Model file for the job. Use its own axes, mm. Face numbers are marked on the shaded views. A direction names the side the tool comes from. Round coordinates to 2 decimals unless told otherwise and drop trailing zeros. Loops run counter-clockwise (first coordinate to the right, second up) from the corner with the lowest first, then second, coordinate; pieces in that order, holes last. Notation, with made-up numbers: M 46.25,48.25 L 78.25,48.25 A12 cw 78.25,60.25 Z; hole C 22.5,43.25 d5. An arc over 180 degrees is marked long. Use a Markdown table: item, result. Add a question column.
Q1. Probe line 1 (X direction, y = 10.5, z = -6.25) (3 decimals); line 2 (Y direction, x = 10.5, z = 5.25) (3 decimals); line 3 (Y direction, x = -18.5, z = 3.25) (3 decimals). List the from-to ranges inside material, lowest first. Write a range as from..to.
Q2. Cut at D-D (y = -11.5). Give the cut face in (x, z) (1 decimal), plus the area to 3 significant figures.
Q3. Mould opens along X. For the marked faces 3, 4, 5 and 6 say: +X half, -X half, draft (parallel to the pull), parting line (faces both ways), or undercut.
Q4. Tool access for the marked faces 1 and 2: list every direction of +Z, -Z, +X, -X, +Y, -Y with a clear straight run to the whole face (end or side of a thin tool).
Q5. Cut at C-C (x = 0). Give the cut face in (y, z) (1 decimal), plus the area to 3 significant figures.
Q6. Cut at B-B (x = -13). Give the cut face in (y, z) (1 decimal), plus the area to 3 significant figures.
Q7. Cut at A-A (z = 0). State how many separate pieces and enclosed holes the cut face has, plus the area to 3 significant figures.
Q8. Pin check, flat tips, straight feed: pin 1 (1.9 mm diameter, centred on x = 0, z = 0, fed in from +Y); pin 2 (3 mm diameter, centred on x = -15.875, z = 0, fed in from +Y); pin 3 (4 mm diameter, centred on x = 0, z = 0, fed in from +Y) (3 decimals); pin 4 (6 mm diameter, centred on x = 22, y = -38, fed in from +Z). Stop position of each tip, or through.
from build123d import *

# Parameters (mm, degrees)
F0_W      = 34.925
F0_H      = 52.705
F1_DEPTH  = 10.795
F2_DEPTH  = 10.795
F3_W      = 25.781
F3_H      = 43.18
F3_H_2    = 36.83
F4_DEPTH  = 25.4
F5_R      = 8.255
F6_W      = 34.925
F6_H      = 19.05
F7_DEPTH  = 5.08
F8_R      = 1.5875
F9_DEPTH  = 50.8
F10_R     = 7.493
F11_DEPTH = 76.2
F12_R     = 8.001
F13_R     = 1.5875
F14_DEPTH = 25.4
F15_SIZE  = 0.762
F16_R     = 2.54
F17_SIZE  = 0.8255
F19_W     = 73.3495355977
F19_H     = 43.3503502247
F20_DEPTH = 25.4
F21_R     = 1.5875
F22_DEPTH = 25.4


with BuildPart() as f1:
    # F0 (on Top) → F1 (new body)
    with BuildSketch(Plane.XY):
        with Locations((-17.4625, -26.3525)):
            Rectangle(F0_W, F0_H)
        with Locations((-17.4625, 26.3525)):
            Rectangle(F0_W, F0_H)
        Polygon((0, 52.705), (0, 0), (0, -52.705), (34.925, -52.705), (34.925, 0), (34.925, 52.705), align=None)
    extrude(amount=F1_DEPTH)

    # F0 (on Top) → F2 (join)
    with BuildSketch(Plane.XY):
        with Locations((-17.4625, -26.3525)):
            Rectangle(F0_W, F0_H)
        with Locations((-17.4625, 26.3525)):
            Rectangle(F0_W, F0_H)
        Polygon((0, 52.705), (0, 0), (0, -52.705), (34.925, -52.705), (34.925, 0), (34.925, 52.705), align=None)
    extrude(amount=-F2_DEPTH)

    # F3 (on face) → F4 (cut)
    with BuildSketch(Plane.XY.offset(10.795)):
        with Locations((-12.8905, -21.59)):
            Rectangle(F3_W, F3_H)
        with Locations((-12.8905, 18.415)):
            Rectangle(F3_W, F3_H_2)
        with Locations((12.8905, -21.59)):
            Rectangle(F3_W, F3_H)
        with Locations((12.8905, 18.415)):
            Rectangle(F3_W, F3_H_2)
    extrude(amount=-F4_DEPTH, mode=Mode.SUBTRACT)

    # F5
    f5_edges = [f1.edges().sort_by_distance(p)[0] for p in [
        (-25.781, 36.83, 0),
        (25.781, 36.83, 0),
        (-25.781, -43.18, 0),
        (25.781, -43.18, 0),
    ]]
    fillet(f5_edges, radius=F5_R)

    # F6 (on face) → F7 (join)
    with BuildSketch(Plane(origin=(0, 52.705, 0), x_dir=(-1, 0, 0), z_dir=(0, 1, 0))):
        Polygon((-34.925, 0), (0, 0), (0, -19.05), (34.925, -19.05), (34.925, 0), (34.925, 19.05), (0, 19.05), (-34.925, 19.05), align=None)
        with Locations((-17.4625, -9.525)):
            Rectangle(F6_W, F6_H)
    extrude(amount=-F7_DEPTH)

    # F8 (on face) → F9 (cut)
    with BuildSketch(Plane.XZ.offset(-47.625)):
        with Locations((22.225, 15.24)):
            Circle(F8_R)
        with Locations((0, 15.24)):
            Circle(F8_R)
        with Locations((0, -15.24)):
            Circle(F8_R)
        with Locations((22.225, -15.24)):
            Circle(F8_R)
        with Locations((-22.225, 15.24)):
            Circle(F8_R)
        with Locations((-22.225, -15.24)):
            Circle(F8_R)
    extrude(amount=-F9_DEPTH, mode=Mode.SUBTRACT)

    # F10 (on face) → F11 (cut)
    with BuildSketch(Plane(origin=(-34.925, 0, 0), x_dir=(0, -1, 0), z_dir=(-1, 0, 0))):
        with Locations((-52.705, 0)):
            Circle(F10_R)
    extrude(amount=-F11_DEPTH, mode=Mode.SUBTRACT)

    # F12
    f12_edges = [f1.edges().sort_by_distance(p)[0] for p in [
        (34.925, -52.705, 0),
        (-34.925, -52.705, 0),
    ]]
    fillet(f12_edges, radius=F12_R)

    # F13 (on face) → F14 (cut)
    with BuildSketch(Plane(origin=(0, 52.705, 0), x_dir=(-1, 0, 0), z_dir=(0, 1, 0))):
        Circle(F13_R)
        with Locations((-15.875, 0)):
            Circle(F13_R)
        with Locations((15.875, 0)):
            Circle(F13_R)
    extrude(amount=-F14_DEPTH, mode=Mode.SUBTRACT)

    # F15
    f15_edges = [f1.edges().sort_by_distance(p)[0] for p in [
        (17.4625, 45.212, 0),
        (1.5875, 45.212, 0),
        (-14.2875, 45.212, 0),
    ]]
    chamfer(f15_edges, length=F15_SIZE)

    # F16
    f16_edges = [f1.edges().sort_by_distance(p)[0] for p in [
        (0, 47.625, -10.795),
        (0, 47.625, 10.795),
    ]]
    fillet(f16_edges, radius=F16_R)

    # F17
    f17_edges = [f1.edges().sort_by_distance(p)[0] for p in [
        (25.781, -3.175, 10.795),
        (34.925, 0.1905, 10.795),
        (34.925, 0.1905, -10.795),
        (25.781, -3.175, -10.795),
        (0, 47.625, -19.05),
        (0, 47.625, 19.05),
    ]]
    chamfer(f17_edges, length=F17_SIZE)

    # F19 (on offset) → F20 (cut)
    with BuildSketch(Plane.XZ.offset(-42.545)):
        with Locations((-0.421330399, -0.413473639)):
            Rectangle(F19_W, F19_H)
    extrude(amount=-F20_DEPTH, mode=Mode.SUBTRACT)

    # F21 (on face) → F22 (cut)
    with BuildSketch(Plane.XZ.offset(52.705)):
        Circle(F21_R)
    extrude(amount=-F22_DEPTH, mode=Mode.SUBTRACT)


solid = f1.part
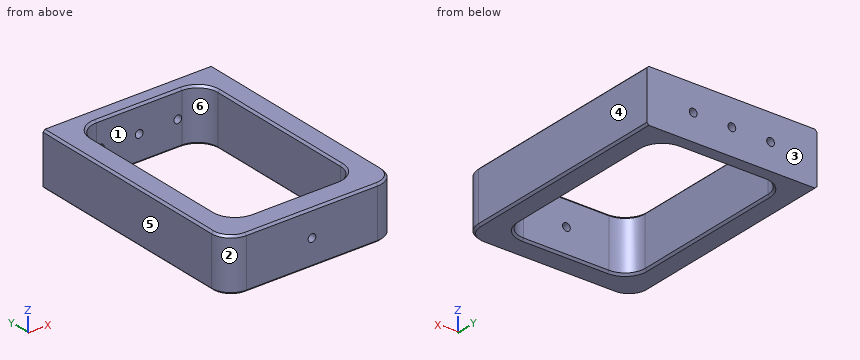
Checked values:
| question | item | result |
|---|---|---|
| 1 | line 1 | x = -34.925..-25.781, 25.781..34.925 |
| 1 | line 2 | y = -52.705..-43.18, 36.83..42.545 |
| 1 | line 3 | y = -52.705..-43.122, 36.772..42.545 |
| 2 | outline | M -34.9,-10 L -34.1,-10.8 L -26.6,-10.8 L -25.8,-10 L -25.8,10 L -26.6,10.8 L -34.1,10.8 L -34.9,10 Z; M 25.8,-10 L 26.6,-10.8 L 34.1,-10.8 L 34.9,-10 L 34.9,10 L 34.1,10.8 L 26.6,10.8 L 25.8,10 Z |
| 2 | area | 392 mm^2 |
| 3 | face 3 | draft |
| 3 | face 4 | +X half |
| 3 | face 5 | -X half |
| 3 | face 6 | undercut |
| 4 | face 1 | +Z, -Z |
| 4 | face 2 | +Z, -Z, -X, -Y |
| 5 | outline | M -52.7,-10 L -51.9,-10.8 L -44,-10.8 L -43.2,-10 L -43.2,-1.6 L -52.7,-1.6 Z; M -52.7,1.6 L -43.2,1.6 L -43.2,10 L -44,10.8 L -51.9,10.8 L -52.7,10 Z; M 36.8,-10 L 37.7,-10.8 L 42.5,-10.8 L 42.5,-1.6 L 36.8,-1.6 Z; M 36.8,1.6 L 42.5,1.6 L 42.5,10.8 L 37.7,10.8 L 36.8,10 Z |
| 5 | area | 279 mm^2 |
| 6 | outline | M -52.7,-10 L -51.9,-10.8 L -44,-10.8 L -43.2,-10 L -43.2,10 L -44,10.8 L -51.9,10.8 L -52.7,10 Z; M 36.8,-10 L 37.7,-10.8 L 42.5,-10.8 L 42.5,10.8 L 37.7,10.8 L 36.8,10 Z |
| 6 | area | 327 mm^2 |
| 7 | separate pieces | 4 |
| 7 | enclosed holes | 0 |
| 7 | area | 2,470 mm^2 |
| 8 | pin 1 | passes through |
| 8 | pin 2 | stops at y = -43.18 |
| 8 | pin 3 | stops at y = 42.545 |
| 8 | pin 4 | stops at z = 10.14 |
